Read the model definition and answer for the solid it produces. Units are mm, in the model's axes. Face numbers are marked on the shaded views. A direction names the side the tool comes from. Coordinates: 2 decimals unless noted, no trailing zeros. Write each loop counter-clockwise with the first axis right and the second up, starting at its lowest first coordinate (ties: lowest second). Pieces come first, ordered by that corner, then holes.
(1) Determine the mould class of the marked faces 1, 2 and 3 for opening direction X: pulls with the +X half, pulls with the -X half, needs draft (parallel to the pull), parting line crosses it, or undercut.
(2) The part is cut by section A-A, the plane x = 9.5. Determine the outline of the cut face in (y, z), and give its area (3 significant figures).
(3) Given pin 1 (1 mm diameter, centred on y = -2.5, z = 1.5, fed in from +X); pin 2 (1.5 mm diameter, centred on y = -1.5, z = 2.5, fed in from +X), each flat-ended and moving along its own axis, determine where each tip first touches the part or whether it passes through.
(4) Which of the six approach directions +Z, -Z, +X, -X, +Y, -Y give full straight-line access (tool end or side, diameter ignored) to the marked faces 4 and 5?
(5) Straight lines are drawn through the part: line 1 along Z through (x, y) = (31, -0.5); line 2 along Z through (x, y) = (-33.5, -0.75); line 3 along X through (y, z) = (-6.75, -1). For each, find the intervals that lie inside material, in ascending order.
(6) The part is cut by section B-B, the plane z = 0. Determine the outline of the cut face in (x, y), and give its area (3 significant figures).
```python
from build123d import *

# Parameters (mm, degrees)
F1_DEPTH = 9


with BuildPart() as f1:
    # F0 (on Front) → F1 (new body)
    with BuildSketch(Plane.XZ):
        with BuildLine():
            ThreePointArc((31.333461, -11.025016), (42.388194, 0.059319), (31.214828, 11.024057))
            Line((31.214828, 11.024057), (0, 11.024057))
            Line((0, 11.024057), (-31.214828, 11.024057))
            ThreePointArc((-31.214828, 11.024057), (-42.388194, 0.059319), (-31.333461, -11.025016))
            Line((-31.333461, -11.025016), (0, -11.025016))
            Line((0, -11.025016), (31.333461, -11.025016))
        make_face()
        with BuildLine():
            ThreePointArc((31.231488, 9.149051), (40.513297, 0.002619), (31.236725, -9.149125))
            Line((31.236725, -9.149125), (0, -9.149125))
            Line((0, -9.149125), (-31.236725, -9.149125))
            ThreePointArc((-31.236725, -9.149125), (-40.513297, 0.002619), (-31.231488, 9.149051))
            Line((-31.231488, 9.149051), (0, 9.149051))
            Line((0, 9.149051), (31.231488, 9.149051))
        make_face(mode=Mode.SUBTRACT)
    extrude(amount=F1_DEPTH)


solid = f1.part
```
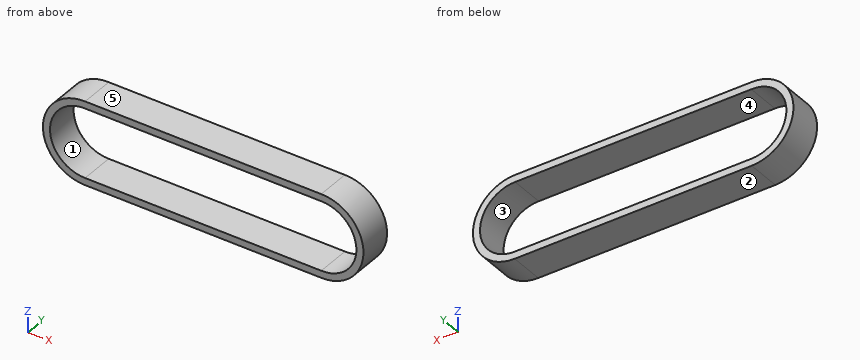
Computed:
1. face 1: undercut
1. face 2: needs draft
1. face 3: undercut
2. outline: (-9, -11.03) - (0, -11.03) - (0, -9.15) - (-9, -9.15) - close; (-9, 9.15) - (0, 9.15) - (0, 11.02) - (-9, 11.02) - close
2. area: 33.8 mm2
3. pin 1: stops at x = 42.34
3. pin 2: stops at x = 42.25
4. face 4: +Y, -Y
4. face 5: +Z, +X, -X, +Y, -Y
5. line 1: z = -11.03 to -9.15, 9.15 to 11.02
5. line 2: z = -10.82 to -8.9, 8.9 to 10.82
5. line 3: x = -42.34 to -40.46, 40.46 to 42.34
6. outline: (-42.39, -9) - (-40.51, -9) - (-40.51, 0) - (-42.39, 0) - close; (40.51, -9) - (42.39, -9) - (42.39, 0) - (40.51, 0) - close
6. area: 33.8 mm2
